Design review of the part built by this model. Coordinates are the model's own, in mm. Face numbers are marked on the shaded views. Give positions to 0.01 mm unless a question says otherwise; leave off trailing zeros. Loops run counter-clockwise (first coordinate to the right, second up) from the corner with the lowest first, then second, coordinate; pieces in that order, holes last. Notation, with made-up numbers: (-5, 19.5) -> (20, 19.5) arc R36 ccw to (20, 56.5) -> close; hole circle Ø6 at (0.25, 70.5). An arc over 180 degrees is marked (long way). Use a Markdown table: item, result. Add a question column.
1. Add section A-A (x = 5.25). State the section outline as (y, z) points, and give its area (3 significant figures).
2. For pin 1 Ø2 at (y, z) = (2, -22.5) entering from +X; pin 2 Ø1.4 at (x, y) = (3, 3.5) entering from -Z; pin 3 Ø1.5 at (y, z) = (1, -6.5) entering from -X; pin 4 Ø0.8 at (y, z) = (2.5, -62.5) entering from +X, all flat-tipped, find the tip position at first contact; note any pin that passes through.
3. To check wall thickness, follow line 1 (Z direction, x = 2, y = 0.95); line 2 (X direction, y = 1.9, z = -20.5); line 3 (X direction, y = 3.95, z = -59.5). State the ranges of each line that lie inside material, in increasing order.
4. Add section D-D (z = -55.5). State the section outline as (x, y) points, and give its area (3 significant figures).
5. Add section B-B (y = 3.5). State the section outline as (x, z) points.
6. Add section C-C (x = 2.75). State the section outline as (y, z) points.
7. Draft analysis for pull direction Z (two halves, no side actions). For the marked faces 1, 2 and 3, state which applies: pulls with the +Z half, pulls with the -Z half, needs draft (parallel to the pull), parting line crosses it, or undercut.
Autodesk Inventor part; units mm, degrees
ref_plane "YZ Plane" through (0, 0, 0) normal (1, 0, 0) x (0, 1, 0)
ref_plane "XZ Plane" through (0, 0, 0) normal (0, 1, 0) x (-1, 0, 0)
ref_plane "XY Plane" through (0, 0, 0) normal (0, 0, 1) x (1, 0, 0)
sketch "Sketch1" plane through (0, 0, 0) normal (0, 1, 0) x (-1, 0, 0)
  line L0 (0, 0) -> (0, -61.8744)
  line L1 (0, 0) -> (-3.4036, 0)
  line L2 (0, -61.8744) -> (-3.4036, -61.8744)
  line L3 (-3.4036, 0) -> (-6.5786, -15.5321)
  line L4 (-6.5786, -15.5321) -> (-3.4036, -31.0642)
  line L5 (-3.4036, -31.0642) -> (-6.5786, -46.3423)
  line L6 (-6.5786, -46.3423) -> (-3.4036, -61.8744)
  dimension "d0" = 61.8744
  dimension "d1" = 3.4036
  dimension "d2" = 3.4036
  dimension "d3" = 15.5321
  dimension "d4" = 31.0642
  dimension "d5" = 15.5321
  dimension "d6" = 3.175
  dimension "d7" = 3.175
extrude "Extrusion1" add sketch "Sketch1" along normal blind 5.4769
sketch "Sketch2" plane through (0, 0, 0) normal (0, 0, 1) x (1, 0, 0)
  line L0 (3.4036, 0) -> (0, 0)
  line L1 (0, 5.4769) -> (1.651, 5.4769)
  line L2 (1.651, 5.4769) -> (1.651, 0)
  line L3 (1.651, 0) -> (0, 0)
  line L4 (0, 0) -> (0, 5.4769)
  dimension "d10" = 1.651
sketch "Sketch3" plane through (3.4036, 0, -61.8744) normal (0, 0, -1) x (-1, 0, 0)
  line L0 (0, 0) -> (3.4036, 0)
  line L1 (3.4036, 5.4769) -> (1.7526, 5.4769)
  line L2 (1.7526, 5.4769) -> (1.7526, 0)
  line L3 (1.7526, 0) -> (3.4036, 0)
  line L4 (3.4036, 0) -> (3.4036, 5.4769)
  dimension "d11" = 1.651
extrude "Extrusion2" add sketch "Sketch3" along normal blind 2.5654
extrude "Extrusion3" add sketch "Sketch2" along normal blind 2.5654
properties part number "Short_insert_CPY1_CPY"
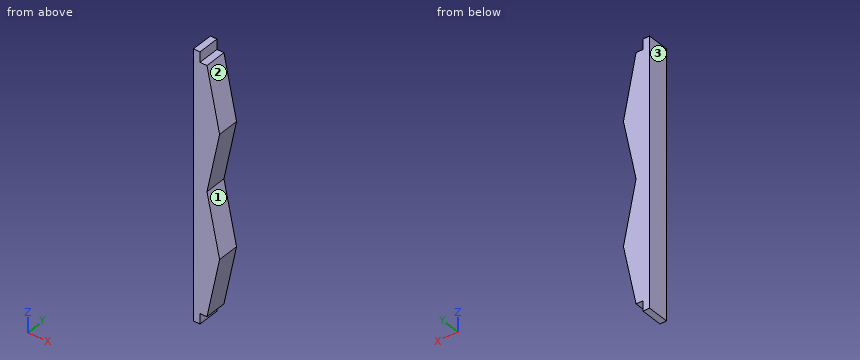
Taken from the geometry:
| question | item | result |
|---|---|---|
| 1 | outline | (0, -52.84) -> (5.48, -52.84) -> (5.48, -39.95) -> (0, -39.95) -> close; (0, -22.03) -> (5.48, -22.03) -> (5.48, -9.03) -> (0, -9.03) -> close |
| 1 | area | 142 mm^2 |
| 2 | pin 1 | stops at x = 5.36 |
| 2 | pin 2 | stops at z = -61.87 |
| 2 | pin 3 | stops at x = 0 |
| 2 | pin 4 | stops at x = 1.65 |
| 3 | line 1 | z = -61.87 to 0 |
| 3 | line 2 | x = 0 to 5.56 |
| 3 | line 3 | x = 0 to 3.89 |
| 4 | outline | (0, 0) -> (4.71, 0) -> (4.71, 5.48) -> (0, 5.48) -> close |
| 4 | area | 25.8 mm^2 |
| 5 | outline | (0, -64.44) -> (1.65, -64.44) -> (1.65, -61.87) -> (3.4, -61.87) -> (6.58, -46.34) -> (3.4, -31.06) -> (6.58, -15.53) -> (3.4, 0) -> (1.65, 0) -> (1.65, 2.57) -> (0, 2.57) -> close |
| 6 | outline | (0, -61.87) -> (5.48, -61.87) -> (5.48, 0) -> (0, 0) -> close |
| 7 | face 1 | undercut |
| 7 | face 2 | pulls with the +Z half |
| 7 | face 3 | needs draft |
